The listing builds one solid part. Answer for the finished solid, in the listing's coordinates (mm). A direction names the side the tool comes from. Give positions to 0.01 mm unless a question says otherwise; leave off trailing zeros. Order: outer loops, then holes, each group sorted by start corner. A loop starts at its lowest first (then second) coordinate and runs counter-clockwise, first axis right, second up.
```python
from build123d import *

# Parameters (mm, degrees)
SKETCH1_W                 = 28.575
SKETCH1_H                 = 38.1
BASE_FLANGE1_DEPTH        = 3.175
EDGE_FLANGE1_DEPTH        = 38.1
BREAK_CORNER1_START       = 42.656216575
BREAK_CORNER1_OUTLINE_W   = 32
BREAK_CORNER1_OUTLINE_H   = 6
BREAK_CORNER1_DEPTH       = 4.490128061
BREAK_CORNER1_START_2     = 15.715448212
BREAK_CORNER1_2_OUTLINE_W = 32
BREAK_CORNER1_2_OUTLINE_H = 6
BREAK_CORNER1_2_DEPTH     = 4.49012806
BREAK_CORNER1_START_3     = 90.251574017
BREAK_CORNER1_3_OUTLINE_W = 6
BREAK_CORNER1_3_OUTLINE_H = 32
BREAK_CORNER1_3_DEPTH     = 4.49012806
BREAK_CORNER1_START_4     = -67.800933714
BREAK_CORNER1_4_OUTLINE_W = 6
BREAK_CORNER1_4_OUTLINE_H = 31
BREAK_CORNER1_4_DEPTH     = 4.49012806
CUT_EXTRUDE1_REACH        = 110.171
CUT_EXTRUDE2_REACH        = 109.061
SKETCH10_R                = 1.5875


# Read off the part's stored shape, not the designer's step: Break-Corner1
# Sheet-metal steps are written as plain solids
with BuildPart() as part:
    # Sketch1 → Base-Flange1 (new body)
    with BuildSketch(Plane.XY):
        with Locations((14.2875, 19.05)):
            Rectangle(SKETCH1_W, SKETCH1_H)
    extrude(amount=-BASE_FLANGE1_DEPTH)

    # Edge-Flange1 section (across the edge) → Edge-Flange1 (add)
    with BuildSketch(Plane(origin=(-0.7366, 38.1, 0), x_dir=(1, 0, 0), z_dir=(0, -1, 0))):
        with BuildLine():
            Line((-3.175, 0.7366), (-3.175, 95.885))
            Line((-3.175, 95.885), (0, 95.885))
            Line((0, 95.885), (0, 0.7366))
            ThreePointArc((0, 0.7366), (0.215745145, 0.215745145), (0.7366, 0))
            Line((0.7366, 0), (0.7366, -3.175))
            ThreePointArc((0.7366, -3.175), (-2.029318885, -2.029318885), (-3.175, 0.7366))
        make_face()
    extrude(amount=EDGE_FLANGE1_DEPTH)

    # Break-Corner1 outline → Break-Corner1 (cut)
    with BuildSketch(Plane(origin=(0, 0, 0), x_dir=(0.707106781186548, -0.707106781186547, 0), z_dir=(0.707106781186547, 0.707106781186548, 0)).offset(BREAK_CORNER1_START)):
        with Locations((3, 2)):
            Rectangle(BREAK_CORNER1_OUTLINE_W, BREAK_CORNER1_OUTLINE_H)
    extrude(amount=BREAK_CORNER1_DEPTH, mode=Mode.SUBTRACT)

    # Break-Corner1 2 outline → Break-Corner1 2 (cut)
    with BuildSketch(Plane(origin=(0, 0, 0), x_dir=(0.707106781186548, 0.707106781186547, 0), z_dir=(0.707106781186547, -0.707106781186548, 0)).offset(BREAK_CORNER1_START_2)):
        with Locations((30, -2)):
            Rectangle(BREAK_CORNER1_2_OUTLINE_W, BREAK_CORNER1_2_OUTLINE_H)
    extrude(amount=BREAK_CORNER1_2_DEPTH, mode=Mode.SUBTRACT)

    # Break-Corner1 3 outline → Break-Corner1 3 (cut)
    with BuildSketch(Plane(origin=(0, 0, 0), x_dir=(1, 0, 0), z_dir=(0, 0.707106781186548, 0.707106781186547)).offset(BREAK_CORNER1_START_3)):
        with Locations((-2, -51)):
            Rectangle(BREAK_CORNER1_3_OUTLINE_W, BREAK_CORNER1_3_OUTLINE_H)
    extrude(amount=BREAK_CORNER1_3_DEPTH, mode=Mode.SUBTRACT)

    # Break-Corner1 4 outline → Break-Corner1 4 (cut)
    with BuildSketch(Plane(origin=(0, 0, 0), x_dir=(1, 0, 0), z_dir=(0, 0.707106781186548, -0.707106781186547)).offset(BREAK_CORNER1_START_4)):
        with Locations((-2, -77.5)):
            Rectangle(BREAK_CORNER1_4_OUTLINE_W, BREAK_CORNER1_4_OUTLINE_H)
    extrude(amount=BREAK_CORNER1_4_DEPTH, mode=Mode.SUBTRACT)

    # Sketch9 → Cut-Extrude1 (cut, up to next)
    with BuildSketch(Plane.ZY.offset(3.9116), mode=Mode.PRIVATE) as cut_extrude1_sk1:
        with BuildLine():
            Line((42.037, 8.636), (78.105, 8.636))
            ThreePointArc((78.105, 8.636), (79.901051224, 9.379948776), (80.645, 11.176))
            Line((80.645, 11.176), (80.645, 26.924))
            ThreePointArc((80.645, 26.924), (79.901051224, 28.720051224), (78.105, 29.464))
            Line((78.105, 29.464), (42.037, 29.464))
            ThreePointArc((42.037, 29.464), (40.240948776, 28.720051224), (39.497, 26.924))
            Line((39.497, 26.924), (39.497, 11.176))
            ThreePointArc((39.497, 11.176), (40.240948776, 9.379948776), (42.037, 8.636))
        make_face()
    cut_extrude1_tool1 = extrude(cut_extrude1_sk1.sketch, amount=-CUT_EXTRUDE1_REACH, mode=Mode.PRIVATE) & part.part
    add(cut_extrude1_tool1.solids().sort_by_distance((-3.9116, 19.05, 60.071))[0], mode=Mode.SUBTRACT)

    # Sketch10 → Cut-Extrude2 (cut, up to next)
    with BuildSketch(Plane.XY, mode=Mode.PRIVATE) as cut_extrude2_sk1:
        with Locations((7.62, 30.96264399)):
            Circle(SKETCH10_R)
    cut_extrude2_tool1 = extrude(cut_extrude2_sk1.sketch, amount=-CUT_EXTRUDE2_REACH, mode=Mode.PRIVATE) & part.part
    # Sketch10 → Cut-Extrude2 (cut, up to next)
    with BuildSketch(Plane.XY, mode=Mode.PRIVATE) as cut_extrude2_sk2:
        with Locations((20.955, 20.183863844)):
            Circle(SKETCH10_R)
    cut_extrude2_tool2 = extrude(cut_extrude2_sk2.sketch, amount=-CUT_EXTRUDE2_REACH, mode=Mode.PRIVATE) & part.part
    # Sketch10 → Cut-Extrude2 (cut, up to next)
    with BuildSketch(Plane.XY, mode=Mode.PRIVATE) as cut_extrude2_sk3:
        with Locations((7.62, 9.405083697)):
            Circle(SKETCH10_R)
    cut_extrude2_tool3 = extrude(cut_extrude2_sk3.sketch, amount=-CUT_EXTRUDE2_REACH, mode=Mode.PRIVATE) & part.part
    add(cut_extrude2_tool1.solids().sort_by_distance((7.62, 30.962644, 0))[0], mode=Mode.SUBTRACT)
    add(cut_extrude2_tool2.solids().sort_by_distance((20.955, 20.183864, 0))[0], mode=Mode.SUBTRACT)
    add(cut_extrude2_tool3.solids().sort_by_distance((7.62, 9.405084, 0))[0], mode=Mode.SUBTRACT)


solid = part.part
```
1) Find section B-B (y = 24.5). Write down the section's boundary in (x, z) (3 decimals), then the cut area to 3 significant figures.
Geometry says:
outline: (-3.912, 0.737) arc R3.912 ccw to (0, -3.175) - (28.575, -3.175) - (28.575, 0) - (0, 0) arc R0.737 cw to (-0.737, 0.737) - (-0.737, 39.497) - (-3.912, 39.497) - close; (-3.912, 80.645) - (-0.737, 80.645) - (-0.737, 95.885) - (-3.912, 95.885) - close
area: 274 mm2
2) Given P1, Ø19, axis at y = 24, z = 51.5, coming from the +X side; P2, Ø2, axis at x = 0.5, z = 63, coming from the -Y side; P3, Ø2.5, axis at x = -3, y = 17.5, coming from the -Z side, each flat-ended and moving along its own axis, determine where each tip first touches the part or whether it passes through.
Geometry says:
P1: stops at x = -0.74
P2: passes through
P3: stops at z = -2.76
3) A tool of negligible diameter and unlimited length cuts with its end or side. For faces 4 (the cylindrical face through (6.45, 10.48, -1.57)), 5 (the cylindrical face through (-2.35, 9.4, 40.22)), 6 (the flat face through (14, 19, 0)), from which of +Z, -Z, +X, -X, +Y, -Y can it reach the whole face along a straight path? Write none if from no direction.
Geometry says:
face 4: +Z, -Z
face 5: +X, -X
face 6: +Z, +X, +Y, -Y
4) For a pull along Y with two mould halves and no side action, classify faces 1 (the cylindrical face through (7.28, 29.41, -1.57)), 2 (the flat face through (25.356, 3.131, -1.565)), 3 (the flat face through (25.356, 34.969, -1.61)) as +Y half, -Y half, draft (parallel to the pull), parting line (faces both ways), or undercut.
Geometry says:
face 1: undercut
face 2: -Y half
face 3: +Y half
5) Straight lines are drawn through the part: probe 1 along Y at (x, z) = (7, -1); probe 2 along Z at (x, y) = (8, 5) (3 decimals); probe 3 along X at (y, z) = (11.5, 86). For each, find the intervals that lie inside material, in ascending order.
Geometry says:
probe 1: y = 0 to 7.94, 10.87 to 29.5, 32.42 to 38.1
probe 2: z = -3.175 to 0
probe 3: x = -3.91 to -0.74
6) Find section C-C (z = 49.5). Write down the section's boundary in (x, y), then the cut area to 3 significant figures.
Geometry says:
outline: (-3.91, 0) - (-0.74, 0) - (-0.74, 8.64) - (-3.91, 8.64) - close; (-3.91, 29.46) - (-0.74, 29.46) - (-0.74, 38.1) - (-3.91, 38.1) - close
area: 54.8 mm2
7) Find section A-A (x = 7.62). Write down the section's boundary in (y, z) (3 decimals), then the cut area to 3 significant figures.
Geometry says:
outline: (0, -3.175) - (7.818, -3.175) - (7.818, 0) - (0, 0) - close; (10.993, -3.175) - (29.375, -3.175) - (29.375, 0) - (10.993, 0) - close; (32.55, -3.175) - (38.1, -3.175) - (38.1, 0) - (32.55, 0) - close
area: 101 mm2
8) Find section D-D (y = 5). Write down the section's boundary in (x, z) (3 decimals).
Geometry says:
outline: (-3.912, 0.737) arc R3.912 ccw to (0, -3.175) - (27.225, -3.175) - (27.225, 0) - (0, 0) arc R0.737 cw to (-0.737, 0.737) - (-0.737, 94.535) - (-3.912, 94.535) - close
